Drawing for the job (mm, zero at the part's lowest x, y, z). Coordinates: 2 decimals unless noted, no trailing zeros. Write each loop counter-clockwise with the first axis right and the second up, starting at its lowest first coordinate (ties: lowest second). Pieces come first, ordered by that corner, then holes. Notation, with made-up numbers: (-3, 66.5) -> (24, 66.5) arc R28 cw to (24, 86.5) -> close; hole circle Ø5 at (-28, 74.25). An arc over 180 degrees is marked (long way). Answer as CSV lines item,"result". Start each with the question number.
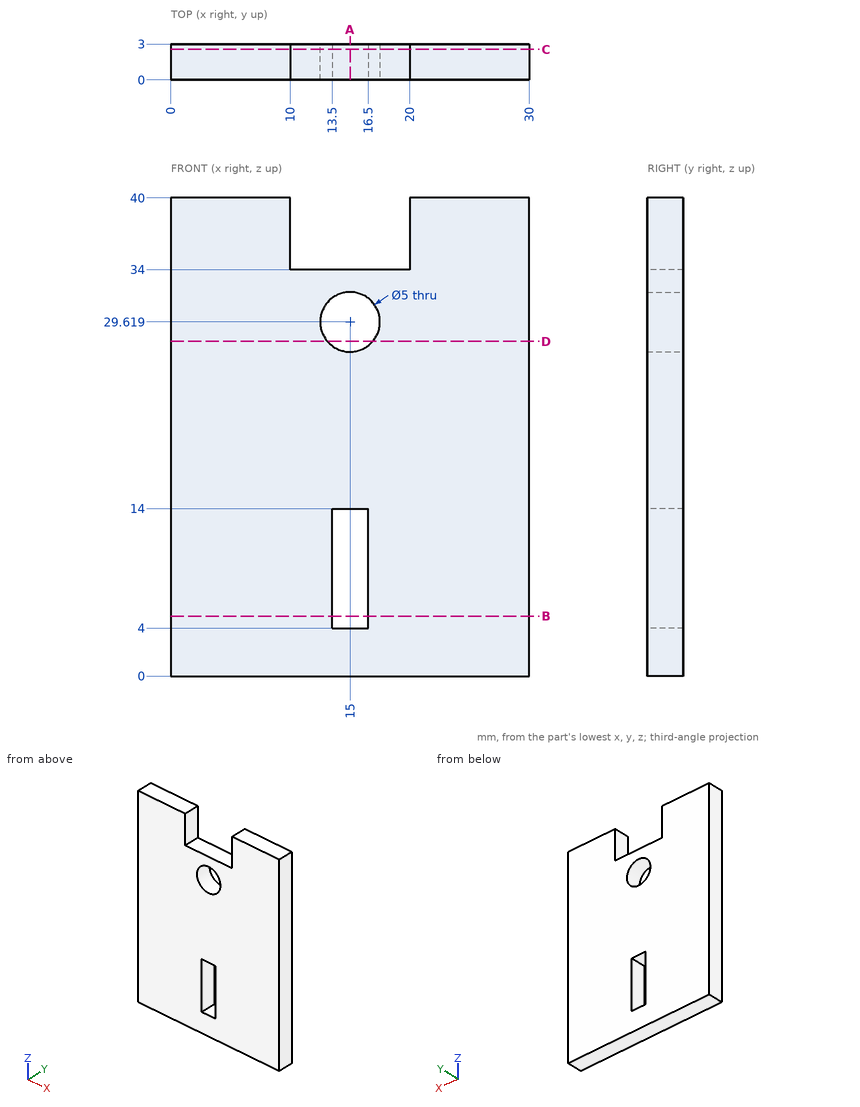
1. Wall check: line 1 (Z direction, x = 15, y = 1.3); line 2 (X direction, y = 2.1, z = 11.5); line 3 (X direction, y = 1.9, z = 37). Give the ranges that are in metal, low to high.
2. Flat gauge pin, fed straight in: P1, Ø4, axis at x = 24, z = 29, coming from the -Y side. Where does the tip first touch, or does it go through?
3. Cut at C-C (y = 2.55). Give the cut face in (x, z).
4. Cut at B-B (z = 5). Give the cut face in (x, y).
5. Cut at A-A (x = 15). Give the cut face in (y, z).
6. Cut at D-D (z = 28). Give the cut face in (x, y) (1 decimal).
Geometry check:
1,line 1,"0 to 4, 14 to 27.12, 32.12 to 34"
1,line 2,"0 to 13.5, 16.5 to 30"
1,line 3,"0 to 10, 20 to 30"
2,P1,"y = 0"
3,outline,"(0, 0) -> (30, 0) -> (30, 40) -> (20, 40) -> (20, 34) -> (10, 34) -> (10, 40) -> (0, 40) -> close; hole circle Ø5 at (15, 29.62); hole (13.5, 4) -> (16.5, 4) -> (16.5, 14) -> (13.5, 14) -> close"
4,outline,"(0, 0) -> (13.5, 0) -> (13.5, 3) -> (0, 3) -> close; (16.5, 0) -> (30, 0) -> (30, 3) -> (16.5, 3) -> close"
5,outline,"(0, 0) -> (3, 0) -> (3, 4) -> (0, 4) -> close; (0, 14) -> (3, 14) -> (3, 27.12) -> (0, 27.12) -> close; (0, 32.12) -> (3, 32.12) -> (3, 34) -> (0, 34) -> close"
6,outline,"(0, 0) -> (13.1, 0) -> (13.1, 3) -> (0, 3) -> close; (16.9, 0) -> (30, 0) -> (30, 3) -> (16.9, 3) -> close"
